from build123d import *

# Parameters (mm, degrees)
SKETCH_1_W          = 41
SKETCH_1_H          = 33
EXTRUDE_1_DEPTH     = 2
SKETCH_2_W          = 35
SKETCH_2_H          = 27
EXTRUDE_2_DEPTH     = 2
SKETCH_3_W          = 8
SKETCH_3_H          = 4
CUT_EXTRUDE_1_DEPTH = 5
SKETCH_5_W          = 1.5
SKETCH_5_H          = 5
CUT_EXTRUDE_2_DEPTH = 1


with BuildPart() as part:
    # Эскиз1 → Бобышка-Вытянуть1 (new body)
    with BuildSketch(Plane.XY):
        Rectangle(SKETCH_1_W, SKETCH_1_H)
    extrude(amount=EXTRUDE_1_DEPTH)

    # Эскиз2 → Бобышка-Вытянуть2 (add)
    with BuildSketch(Plane.XY.offset(2)):
        Rectangle(SKETCH_2_W, SKETCH_2_H)
    extrude(amount=EXTRUDE_2_DEPTH)

    # Эскиз3 → Вырез-Вытянуть1 (cut)
    with BuildSketch(Plane.XY.offset(4)):
        with Locations((0, 9)):
            Rectangle(SKETCH_3_W, SKETCH_3_H)
    extrude(amount=-CUT_EXTRUDE_1_DEPTH, mode=Mode.SUBTRACT)

    # Эскиз5 → Вырез-Вытянуть2 (cut)
    with BuildSketch(Plane.XY.offset(2)):
        with Locations((-19.75, 0)):
            Rectangle(SKETCH_5_W, SKETCH_5_H)
        with Locations((19.75, 0)):
            Rectangle(SKETCH_5_W, SKETCH_5_H)
    extrude(amount=-CUT_EXTRUDE_2_DEPTH, mode=Mode.SUBTRACT)


solid = part.part
Can you work these out from the model? Positions are in its coordinate system, mm. A direction names the side the tool comes from. Round coordinates to 2 decimals unless told otherwise and drop trailing zeros. Order: outer loops, then holes, each group sorted by start corner. A loop starts at its lowest first (then second) coordinate and runs counter-clockwise, first axis right, second up. Notation, with made-up numbers: M -23.75,1.5 L -9.75,1.5 A7 cw -9.75,14.5 Z; hole C 40,19 d6. An arc over 180 degrees is marked long. Use a Markdown table: item, result.
1) Imagine slicing it at A-A (x = -0.5). List the corners of the cut face in (y, z) for me.
Geometry says:
| item | result |
|---|---|
| outline | M -16.5,0 L 7,0 L 7,4 L -13.5,4 L -13.5,2 L -16.5,2 Z; M 11,0 L 16.5,0 L 16.5,2 L 13.5,2 L 13.5,4 L 11,4 Z |
2) Imagine slicing it at C-C (y = 13). List the corners of the cut face in (x, z) for me.
Geometry says:
| item | result |
|---|---|
| outline | M -20.5,0 L 20.5,0 L 20.5,2 L 17.5,2 L 17.5,4 L -17.5,4 L -17.5,2 L -20.5,2 Z |
3) On a 3-axis mill with a long thin cutter (end or side, diameter ignored), from which of +Z, -Z, +X, -X, +Y, -Y can I reach the whole of each face in a straight line? I mean faces 5 (the face through (-19.8, 2.5, 1.5)), 6 (the face through (19, 0, 1.5)), 7 (the face through (17.5, 0, 3)), 8 (the face through (0, 11, 2)). Say none if no direction works.
Geometry says:
| item | result |
|---|---|
| face 5 | +Z, -X |
| face 6 | +Z, +X |
| face 7 | +Z, +X, +Y, -Y |
| face 8 | +Z, -Z |
4) Imagine slicing it at D-D (x = -11.5). List the corners of the cut face in (y, z) for me.
Geometry says:
| item | result |
|---|---|
| outline | M -16.5,0 L 16.5,0 L 16.5,2 L 13.5,2 L 13.5,4 L -13.5,4 L -13.5,2 L -16.5,2 Z |
5) If I drill on line 1 along Y through (x, z) = (1, 3.7); line 2 along Z through (x, y) = (-18, -2.5); line 3 along Y through (x, z) = (0.5, 1.15), over which ranges is the centre line in solid material (lowest first)?
Geometry says:
| item | result |
|---|---|
| line 1 | y = -13.5 to 7, 11 to 13.5 |
| line 2 | z = 0 to 2 |
| line 3 | y = -16.5 to 7, 11 to 16.5 |
6) If we mould it in two halves opening along X, with no side actions, what happens to faces 1 (the face through (19.7, 2.5, 1.5)), 2 (the face through (0, 7, 2)), 3 (the face through (4, 9, 2)), 4 (the face through (20.5, -0.2, 0.8))? For each: +X half, -X half, draft (parallel to the pull), parting line (faces both ways), or undercut.
Geometry says:
| item | result |
|---|---|
| face 1 | draft |
| face 2 | undercut |
| face 3 | undercut |
| face 4 | +X half |
7) Imagine slicing it at B-B (z = 3). List the corners of the cut face in (x, y) for me, then the cut area to 3 significant figures.
Geometry says:
| item | result |
|---|---|
| outline | M -17.5,-13.5 L 17.5,-13.5 L 17.5,13.5 L -17.5,13.5 Z; hole M -4,7 L 4,7 L 4,11 L -4,11 Z |
| area | 913 mm² |
8) I'm going to push flat-ended pins straight in: P1, Ø1.5, axis at y = 0.5, z = 3.5, coming from the +X side; P2, Ø1.6, axis at y = 5, z = 3, coming from the -X side. Where does each tip first touch, or does it pass through?
Geometry says:
| item | result |
|---|---|
| P1 | stops at x = 17.5 |
| P2 | stops at x = -17.5 |
